Here's the drawing with two shaded views (mm, measured from the low corner). I have some questions. Round coordinates to 2 decimals unless told otherwise and drop trailing zeros. Order: outer loops, then holes, each group sorted by start corner. A loop starts at its lowest first (then second) coordinate and runs counter-clockwise, first axis right, second up. Notation, with made-up numbers: (70, 77) - (113, 77) arc R25 ccw to (113, 111) - close; hole circle Ø7 at (-19, 48). An arc over 180 degrees is marked (long way). One line per item, written item: value.
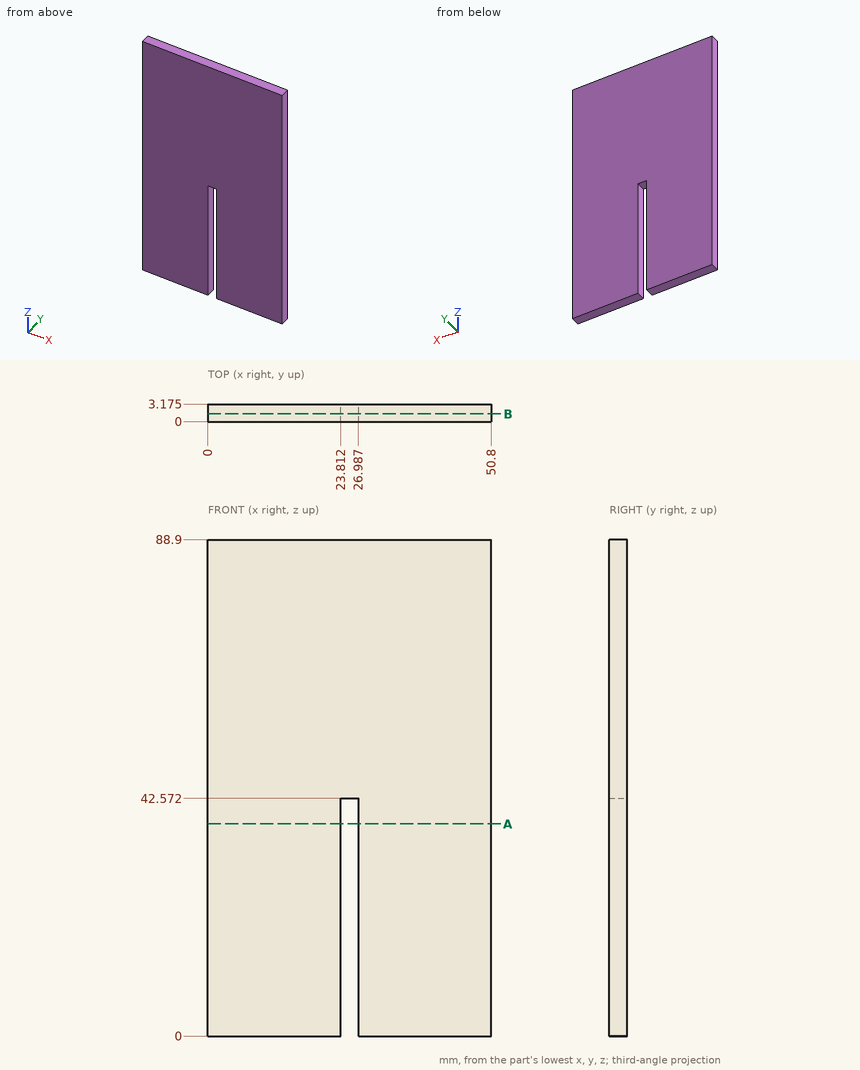
Q1. If we section it at A-A, the plane z = 38: Please give me the cut outline in (x, y) (1 decimal).
Results list:
outline: (0, 0) - (23.8, 0) - (23.8, 3.2) - (0, 3.2) - close; (27, 0) - (50.8, 0) - (50.8, 3.2) - (27, 3.2) - close
Q2. Will this pin go through, and if not, where does the flat tip stop? pin 1 (1.6 mm diameter, centred on x = 25.5, y = 1.5, fed in from -Z).
Results list:
pin 1: z = 42.57
Q3. If we section it at B-B, the plane y = 1.4: Please give me the cut outline in (x, z), then the cut area to 3 significant figures.
Results list:
outline: (0, 0) - (23.81, 0) - (23.81, 42.57) - (26.99, 42.57) - (26.99, 0) - (50.8, 0) - (50.8, 88.9) - (0, 88.9) - close
area: 4,380 mm²
Q4. If I drill on line 1 along X through (y, z) = (2.05, 14); line 2 along Z through (x, y) = (24, 2.3), over which ranges is the centre line in solid material (lowest first)?
Results list:
line 1: 0 to 23.81, 26.99 to 50.8
line 2: 42.57 to 88.9
